Here's how the part is built. I have some questions about the finished solid (model axes, mm). Face numbers are marked on the shaded views. A direction names the side the tool comes from. Round coordinates to 2 decimals unless told otherwise and drop trailing zeros. Write each loop counter-clockwise with the first axis right and the second up, starting at its lowest first coordinate (ties: lowest second). Pieces come first, ordered by that corner, then holes. Notation, with made-up numbers: (57, -35) -> (116, -35) arc R23 cw to (116, -9) -> close; hole circle Ø1 at (54, -17). An arc over 180 degrees is marked (long way). Answer as CSV lines item,"result".
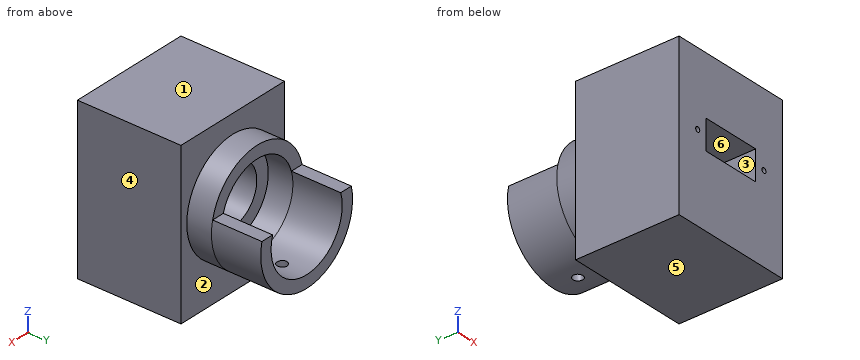
from build123d import *

# Parameters (mm, degrees)
SKETCH023_W     = 25
SKETCH023_H     = 32.5
SKETCH023_R     = 5.8166
PAD011_DEPTH    = 5
SKETCH024_R     = 11.0946
SKETCH024_R_2   = 8.5946
PAD012_DEPTH    = 5
SKETCH025_W     = 25
SKETCH025_H     = 32.5
SKETCH025_R     = 0.5
SKETCH025_W_2   = 12
SKETCH025_H_2   = 6
PAD013_DEPTH    = 16
PAD020_DEPTH    = 10
SKETCH035_R     = 1
POCKET007_DEPTH = 16


with BuildPart() as part:
    # Sketch023 → Pad011 (new body)
    with BuildSketch(Plane.XZ):
        with Locations((0, 6.25)):
            Rectangle(SKETCH023_W, SKETCH023_H)
        with Locations((0, 7.5946)):
            Circle(SKETCH023_R, mode=Mode.SUBTRACT)
    extrude(amount=PAD011_DEPTH)

    # Sketch024 (on Face6 of Pad011) → Pad012 (join)
    with BuildSketch(Plane(origin=(0, 0, 0), x_dir=(1, 0, 0), z_dir=(0, 1, 0))):
        with Locations((0, -7.5946)):
            Circle(SKETCH024_R)
        with Locations((0, -7.5946)):
            Circle(SKETCH024_R_2, mode=Mode.SUBTRACT)
    extrude(amount=PAD012_DEPTH)

    # Sketch025 (on Face5 of Pad012) → Pad013 (join)
    with BuildSketch(Plane.XZ.offset(5)):
        with Locations((0, 6.25)):
            Rectangle(SKETCH025_W, SKETCH025_H)
        with Locations((-8, 7.5946)):
            Circle(SKETCH025_R, mode=Mode.SUBTRACT)
        with Locations((8, 7.5946)):
            Circle(SKETCH025_R, mode=Mode.SUBTRACT)
        with Locations((0, 7.5946)):
            Rectangle(SKETCH025_W_2, SKETCH025_H_2, mode=Mode.SUBTRACT)
    extrude(amount=PAD013_DEPTH)

    # Sketch034 → Pad020 (join)
    with BuildSketch(Plane(origin=(0, 5, 0), x_dir=(1, 0, 0), z_dir=(0, 1, 0))):
        with BuildLine():
            ThreePointArc((8.222965, -10.0946), (0, 1), (-8.222965, -10.0946))
            Line((-10.809262, -10.0946), (-8.222965, -10.0946))
            ThreePointArc((10.809262, -10.0946), (0, 3.5), (-10.809262, -10.0946))
            Line((8.222965, -10.0946), (10.809262, -10.0946))
        make_face()
    extrude(amount=PAD020_DEPTH)

    # Sketch035 → Pocket007 (cut)
    with BuildSketch(Plane.XY):
        with Locations((0, 10)):
            Circle(SKETCH035_R)
    extrude(amount=-POCKET007_DEPTH, mode=Mode.SUBTRACT)


with BuildPart() as part_1:
    # Body005 placement: moved
    add(part.part.moved(Location((0, -373, 0))))


solid = part_1.part
Item 1: Suppose I cut it at D-D, the plane y = -363. List the corners of the cut face in (x, z) for me, then the cut area to 3 significant figures.
Results found:
outline,"(-10.81, 10.09) arc R11.09 ccw to (-1, -3.45) -> (-1, -0.94) arc R8.59 cw to (-8.22, 10.09) -> close; (1, -3.45) arc R11.09 ccw to (10.81, 10.09) -> (8.22, 10.09) arc R8.59 cw to (1, -0.94) -> close"
area,"85.0 mm²"
Item 2: Will these pins go through, and if not, where does the flat tip stop? pin 1 (2 mm diameter, centred on x = -1.5, z = 15, fed in from +Y); pin 2 (0.8 mm diameter, centred on x = -5.5, z = 9, fed in from -Y); pin 3 (2 mm diameter, centred on x = 6.5, y = -368, fed in from -Z).
Results found:
pin 1,"stops at y = -373"
pin 2,"stops at y = -378"
pin 3,"stops at z = -2.04"
Item 3: For the marked faces 1, 2 and 3, which set-ups out of +Z, -Z, +X, -X, +Y, -Y let a thin tool reach every point of the face, with its end or its side?
Results found:
face 1,"+Z, +X, -X, +Y, -Y"
face 2,"+Y"
face 3,"-Y"
Item 4: Suppose I cut it at C-C, the plane x = 3.75. List the corners of the cut face in (y, z) for me, then the cut area to 3 significant figures.
Results found:
outline,"(-394, -10) -> (-373, -10) -> (-373, -2.85) -> (-358, -2.85) -> (-358, -0.14) -> (-373, -0.14) -> (-373, 3.15) -> (-378, 3.15) -> (-378, 4.59) -> (-394, 4.59) -> close; (-394, 10.59) -> (-378, 10.59) -> (-378, 12.04) -> (-373, 12.04) -> (-373, 15.33) -> (-368, 15.33) -> (-368, 18.04) -> (-373, 18.04) -> (-373, 22.5) -> (-394, 22.5) -> close"
area,"596 mm²"
Item 5: I need wall thicknesses on L1, parallel to Z at x = 8, y = -387.5; L2, parallel to Z at x = -2.5, y = -380; L3, parallel to X at y = -381.5, z = 5.5. Which ranges of each line are inside material? Lowest first, please.
Results found:
L1,"z = -10 to 7.09, 8.09 to 22.5"
L2,"z = -10 to 4.59, 10.59 to 22.5"
L3,"x = -12.5 to -6, 6 to 12.5"
Item 6: If we mould it in two halves opening along Z, with no side actions, what happens to the marked faces 4, 5 and 6? For each: pulls with the +Z half, pulls with the -Z half, needs draft (parallel to the pull), parting line crosses it, or undercut.
Results found:
face 4,"needs draft"
face 5,"pulls with the -Z half"
face 6,"undercut"
Item 7: Suppose I cut it at B-B, the plane y = -390. List the corners of the cut face in (x, z) for me, then the cut area to 3 significant figures.
Results found:
outline,"(-12.5, -10) -> (12.5, -10) -> (12.5, 22.5) -> (-12.5, 22.5) -> close; hole circle Ø1 at (-8, 7.59); hole (-6, 4.59) -> (6, 4.59) -> (6, 10.59) -> (-6, 10.59) -> close; hole circle Ø1 at (8, 7.59)"
area,"739 mm²"
Item 8: Suppose I cut it at A-A, the plane x = 0. List the corners of the cut face in (y, z) for me, then the cut area to 3 significant figures.
Results found:
outline,"(-394, -10) -> (-373, -10) -> (-373, -3.5) -> (-364, -3.5) -> (-364, -1) -> (-373, -1) -> (-373, 1.78) -> (-378, 1.78) -> (-378, 4.59) -> (-394, 4.59) -> close; (-394, 10.59) -> (-378, 10.59) -> (-378, 13.41) -> (-373, 13.41) -> (-373, 16.19) -> (-368, 16.19) -> (-368, 18.69) -> (-373, 18.69) -> (-373, 22.5) -> (-394, 22.5) -> close; (-362, -3.5) -> (-358, -3.5) -> (-358, -1) -> (-362, -1) -> close"
area,"573 mm²"
